from build123d import *

# Parameters (mm, degrees)
SKETCH1_R             = 4.9
SKETCH1_R_2           = 2.9
BOSS_EXTRUDE1_DEPTH   = 5
BOSS_EXTRUDE1_2_DEPTH = 5
BOSS_EXTRUDE1_3_DEPTH = 5
BOSS_EXTRUDE1_4_DEPTH = 5
SKETCH3_W             = 80
SKETCH3_H             = 15
BOSS_EXTRUDE2_DEPTH   = 2
SKETCH4_R             = 2.9
CUT_EXTRUDE1_DEPTH    = 42.003048667


with BuildPart() as part:
    # Sketch1 → Boss-Extrude1 (new body)
    with BuildSketch(Plane.XY):
        with Locations((-15.5, 0)):
            Circle(SKETCH1_R)
        with Locations((-15.5, 0)):
            Circle(SKETCH1_R_2, mode=Mode.SUBTRACT)
    extrude(amount=BOSS_EXTRUDE1_DEPTH)



with BuildPart() as body_2:
    # Sketch1 → Boss-Extrude1 2 (new body)
    with BuildSketch(Plane.XY):
        with Locations(Location((-30.5, 0, 0), (0, 0, 180))):
            Circle(SKETCH1_R)
        with Locations(Location((-30.5, 0, 0), (0, 0, 180))):
            Circle(SKETCH1_R_2, mode=Mode.SUBTRACT)
    extrude(amount=BOSS_EXTRUDE1_2_DEPTH)


with BuildPart() as body_3:
    # Sketch1 → Boss-Extrude1 3 (new body)
    with BuildSketch(Plane.XY):
        with Locations(Location((15.5, 0, 0), (0, 0, 180))):
            Circle(SKETCH1_R)
        with Locations(Location((15.5, 0, 0), (0, 0, 180))):
            Circle(SKETCH1_R_2, mode=Mode.SUBTRACT)
    extrude(amount=BOSS_EXTRUDE1_3_DEPTH)


with BuildPart() as body_4:
    # Sketch1 → Boss-Extrude1 4 (new body)
    with BuildSketch(Plane.XY):
        with Locations((30.5, 0)):
            Circle(SKETCH1_R)
        with Locations((30.5, 0)):
            Circle(SKETCH1_R_2, mode=Mode.SUBTRACT)
    extrude(amount=BOSS_EXTRUDE1_4_DEPTH)


with BuildPart() as part_1:
    add(part.part)

    add(body_2.part)  # Boss-Extrude2 merges body 2

    add(body_3.part)  # Boss-Extrude2 merges body 3

    add(body_4.part)  # Boss-Extrude2 merges body 4
    # Sketch3 → Boss-Extrude2 (add)
    with BuildSketch(Plane.XY):
        Rectangle(SKETCH3_W, SKETCH3_H)
    extrude(amount=BOSS_EXTRUDE2_DEPTH)

    # Sketch4 → Cut-Extrude1 (cut, through all)
    with BuildSketch(Plane.XY.offset(5)):
        with Locations(Location((-30.5, 0, 0), (0, 0, 180))):
            Circle(SKETCH4_R)
        with Locations((-15.5, 0)):
            Circle(SKETCH4_R)
        with Locations(Location((15.5, 0, 0), (0, 0, 180))):
            Circle(SKETCH4_R)
        with Locations((30.5, 0)):
            Circle(SKETCH4_R)
    extrude(amount=-CUT_EXTRUDE1_DEPTH, mode=Mode.SUBTRACT)


solid = part_1.part
Geometry: final body of the model. Coordinates: model frame, mm. A direction names the side the tool comes from. Give positions to 0.01 mm unless a question says otherwise; leave off trailing zeros. Order: outer loops, then holes, each group sorted by start corner. A loop starts at its lowest first (then second) coordinate and runs counter-clockwise, first axis right, second up. Notation, with made-up numbers: (70.5, 37) -> (98.5, 37) arc R10 cw to (98.5, 42) -> close; hole circle Ø4 at (63.5, 71.25). An arc over 180 degrees is marked (long way). Put each result on its own line as item: value.
Q1. Section C-C, the plane y = 0. Count the separate pieces of the cut face and the enclosed holes in it, then the cut area to 3 significant figures.
Here are the results:
separate pieces: 5
enclosed holes: 0
area: 162 mm^2
Q2. Section D-D, the plane x = -32. Return loops of the section in (y, z).
Here are the results:
outline: (-7.5, 0) -> (-2.48, 0) -> (-2.48, 5) -> (-4.66, 5) -> (-4.66, 2) -> (-7.5, 2) -> close; (2.48, 0) -> (7.5, 0) -> (7.5, 2) -> (4.66, 2) -> (4.66, 5) -> (2.48, 5) -> close
Q3. Material intervals for L1, parallel to Y at x = -30.5, z = 1.3; L2, parallel to Y at x = -30.5, z = 2.85; L3, parallel to Z at x = 29, y = -6.5, sorted ascending.
Here are the results:
L1: y = -7.5 to -2.9, 2.9 to 7.5
L2: y = -4.9 to -2.9, 2.9 to 4.9
L3: z = 0 to 2
Q4. Section A-A, the plane z = 3. Return loops of the section in (x, y).
Here are the results:
outline: circle Ø9.8 at (-30.5, 0); circle Ø9.8 at (-15.5, 0); circle Ø9.8 at (15.5, 0); circle Ø9.8 at (30.5, 0); hole circle Ø5.8 at (-30.5, 0); hole circle Ø5.8 at (-15.5, 0); hole circle Ø5.8 at (15.5, 0); hole circle Ø5.8 at (30.5, 0)
Q5. Pin query (flat end, axial travel): pin 1 (8 mm diameter, centred on x = -6.5, y = 4.5, fed in from -Z). Return the tip coordinate at first contact, or that it passes through.
Here are the results:
pin 1: stops at z = 0
Q6. Draft query along Y for faces 3 (the face through (-33.266, -0.871, 2.535)), 4 (the face through (-19.39, -2.98, 3.48)), 5 (the face through (13, 2, 5)). Return one class per face: released by +Y, released by -Y, zero draft, split by the parting line, or undercut.
Here are the results:
face 3: undercut
face 4: split by the parting line
face 5: zero draft
Q7. Reachability of faces 1 (the face through (20.395, -0.215, 3.479)), 2 (the face through (-18.4, 0.1, 2.5)) from +Z, -Z, +X, -X, +Y, -Y: full face, straight path, thin tool, end or side. Return the list, or none.
Here are the results:
face 1: +Z
face 2: +Z, -Z
Q8. Section B-B, the plane x = -15.5. Return loops of the section in (y, z), then the cut area to 3 significant figures.
Here are the results:
outline: (-7.5, 0) -> (-2.9, 0) -> (-2.9, 5) -> (-4.9, 5) -> (-4.9, 2) -> (-7.5, 2) -> close; (2.9, 0) -> (7.5, 0) -> (7.5, 2) -> (4.9, 2) -> (4.9, 5) -> (2.9, 5) -> close
area: 30.4 mm^2
